from build123d import *

# Parameters (mm, degrees)
F1_DEPTH = 25
F2_R     = 12.5
F3_DEPTH = 25.001
F4_R     = 12.5
F5_DEPTH = 50


with BuildPart() as f1:
    # F0 (on Top) → F1 (new body)
    with BuildSketch(Plane.XY):
        with BuildLine():
            Line((351.28284, 44.981711), (3.134557, 54.910605))
            Line((3.134557, 54.910605), (0, 55))
            ThreePointArc((0, 55), (-55, 0), (0, -55))
            Line((0, -55), (3.134557, -54.910605))
            Line((3.134557, -54.910605), (351.28284, -44.981711))
            ThreePointArc((351.28284, -44.981711), (395, 0), (351.28284, 44.981711))
        make_face()
    extrude(amount=F1_DEPTH)

    # F2 (on face) → F3 (cut, through all)
    with BuildSketch(Plane.XY.offset(25)):
        Circle(F2_R)
    extrude(amount=-F3_DEPTH, mode=Mode.SUBTRACT)

    # F4 (on face) → F5 (join)
    with BuildSketch(Plane.XY.offset(25)):
        with Locations((350, 0)):
            Circle(F4_R)
    extrude(amount=F5_DEPTH)


solid = f1.part
Geometry check sheet. Reference: the model listing, model coordinates, mm. Give positions to 0.01 mm unless a question says otherwise; leave off trailing zeros. Order: outer loops, then holes, each group sorted by start corner. A loop starts at its lowest first (then second) coordinate and runs counter-clockwise, first axis right, second up.
1) Cross-section at A-A (y = 0). Record the boundary of the cut face in (x, z), then the cut area to 3 significant figures.
Results are:
outline: (-55, 0) - (-12.5, 0) - (-12.5, 25) - (-55, 25) - close; (12.5, 0) - (395, 0) - (395, 25) - (362.5, 25) - (362.5, 75) - (337.5, 75) - (337.5, 25) - (12.5, 25) - close
area: 11,900 mm2
2) Material ranges on probe 1 along Y at (x, z) = (0, 16); probe 2 along Z at (x, y) = (206.5, -44); probe 3 along X at (y, z) = (-26.5, 3), recorded low to high.
Results are:
probe 1: y = -55 to -12.5, 12.5 to 55
probe 2: z = 0 to 25
probe 3: x = -48.19 to 386.37
3) Cross-section at C-C (y = 33.5). Record the boundary of the cut face in (x, z).
Results are:
outline: (-43.62, 0) - (380.05, 0) - (380.05, 25) - (-43.62, 25) - close
4) Cross-section at D-D (x = 201). Record the boundary of the cut face in (y, z), then the cut area to 3 significant figures.
Results are:
outline: (-49.27, 0) - (49.27, 0) - (49.27, 25) - (-49.27, 25) - close
area: 2,460 mm2
5) Cross-section at B-B (z = 40). Record the boundary of the cut face in (x, y), then the cut area to 3 significant figures.
Results are:
outline: circle Ø25 at (350, 0)
area: 491 mm2
6) Gauge pin test, flat ends, axial feed: pin 1 (1 mm diameter, centred on x = 88, y = 7, fed in from -Z); pin 2 (12 mm diameter, centred on x = 161.5, z = 10, fed in from +Y); pin 3 (1 mm diameter, centred on y = 25.5, z = 16.5, fed in from +X); pin 4 (1 mm diameter, centred on x = 298.5, y = 12, fed in from +Z). Record the tip position at first contact, or that the pin passes through.
Results are:
pin 1: stops at z = 0
pin 2: stops at y = 50.57
pin 3: stops at x = 387.42
pin 4: stops at z = 25
7) Draft check along X on faces 1 (the cylindrical face through (361.923, 3.755, 49.65)), 2 (the cylindrical face through (11.923, 3.755, 12.675)), 3 (the flat face through (167, 1, 25)). Enter one of: released by +X, released by -X, zero draft, split by the parting line, or undercut.
Results are:
face 1: split by the parting line
face 2: undercut
face 3: zero draft
